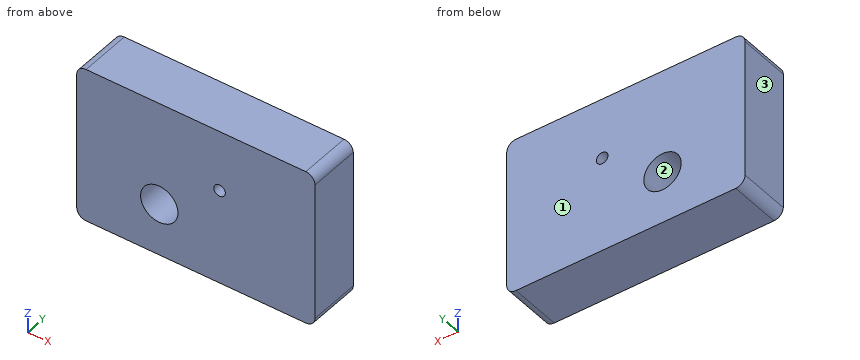
```python
from build123d import *

# Parameters (mm, degrees)
SKETCH1_W           = 27.5
SKETCH1_H           = 18
SKETCH1_R           = 2.25
SKETCH1_R_2         = 0.75
BOSS_EXTRUDE1_DEPTH = 6
FILLET1_R           = 1
MOVE_FACE1_BY       = 0.08
MOVE_FACE1_2_BY     = 0.08
MOVE_FACE1_3_BY     = 0.08
MOVE_FACE1_4_BY     = 0.08
MOVE_FACE1_5_BY     = 0.08
MOVE_FACE1_6_BY     = 0.08
MOVE_FACE1_7_BY     = 0.08
MOVE_FACE1_8_BY     = 0.08
MOVE_FACE1_9_BY     = 0.08
MOVE_FACE1_10_BY    = 0.08


with BuildPart() as part:
    # Sketch1 → Boss-Extrude1 (new body)
    with BuildSketch(Plane(origin=(0, 0, 0), x_dir=(1, 0, 0), z_dir=(0, 1, 0))):
        with Locations((13.75, 9)):
            Rectangle(SKETCH1_W, SKETCH1_H)
        with Locations(Location((9.5, 12, 0), (0, 0, 270))):
            Circle(SKETCH1_R, mode=Mode.SUBTRACT)
        with Locations(Location((16.5, 7, 0), (0, 0, 270))):
            Circle(SKETCH1_R_2, mode=Mode.SUBTRACT)
    extrude(amount=BOSS_EXTRUDE1_DEPTH)

    # Fillet1
    fillet1_edges = [part.edges().sort_by_distance(p)[0] for p in [
        (0, 3, -18),
        (27.5, 3, -18),
        (27.5, 3, 0),
        (0, 3, 0),
    ]]
    fillet(fillet1_edges, radius=FILLET1_R)

    # Move Face1: a curved face moved outward by 0.08
    add(Solid.thicken(part.faces().sort_by_distance((16.5, 3, -7.75))[0], MOVE_FACE1_BY))

    # Move Face1 2: a curved face moved outward by 0.08
    add(Solid.thicken(part.faces().sort_by_distance((9.5, 3, -14.25))[0], MOVE_FACE1_2_BY))

    # Move Face1 3: a curved face moved outward by 0.08
    add(Solid.thicken(part.faces().sort_by_distance((0.292893219, 3, -0.292893219))[0], MOVE_FACE1_3_BY))

    # Move Face1 4: a face moved outward by 0.08
    extrude(part.faces().sort_by_distance((0, 3, -9))[0], amount=MOVE_FACE1_4_BY, dir=(-1, 0, 0))

    # Move Face1 5: a curved face moved outward by 0.08
    add(Solid.thicken(part.faces().sort_by_distance((0.292893219, 3, -17.707106781))[0], MOVE_FACE1_5_BY))

    # Move Face1 6: a face moved outward by 0.08
    extrude(part.faces().sort_by_distance((13.75, 3, -18))[0], amount=MOVE_FACE1_6_BY, dir=(0, 0, -1))

    # Move Face1 7: a curved face moved outward by 0.08
    add(Solid.thicken(part.faces().sort_by_distance((27.207106781, 3, -17.707106781))[0], MOVE_FACE1_7_BY))

    # Move Face1 8: a face moved outward by 0.08
    extrude(part.faces().sort_by_distance((27.5, 3, -9))[0], amount=MOVE_FACE1_8_BY, dir=(1, 0, 0))

    # Move Face1 9: a curved face moved outward by 0.08
    add(Solid.thicken(part.faces().sort_by_distance((27.207106781, 3, -0.292893219))[0], MOVE_FACE1_9_BY))

    # Move Face1 10: a face moved outward by 0.08
    extrude(part.faces().sort_by_distance((13.75, 3, 0))[0], amount=MOVE_FACE1_10_BY, dir=(0, 0, 1))


solid = part.part
```
The listing builds one solid part. Answer for the finished solid, in the listing's coordinates (mm). Face numbers are marked on the shaded views. Give positions to 0.01 mm unless a question says otherwise; leave off trailing zeros. Write each loop counter-clockwise with the first axis right and the second up, starting at its lowest first coordinate (ties: lowest second). Pieces come first, ordered by that corner, then holes. Notation, with made-up numbers: (73, -34.5) -> (116, -34.5) arc R9 ccw to (116, -26.5) -> close; hole circle Ø1 at (36.25, -17.5). An arc over 180 degrees is marked (long way). Write item = value, one per line. Start each with the question number.
1) Determine the mould class of the marked faces 1, 2 and 3 for opening direction X: +X half, -X half, draft (parallel to the pull), parting line (faces both ways), or undercut.
2) The part is cut by section A-A, the plane z = -7. Determine the outline of the cut face in (x, y), and give its area (3 significant figures).
3) The part is cut by section B-B, the plane y = 3.25. Determine the outline of the cut face in (x, z), and give its area (3 significant figures).
4) Straight lines are drawn through the part: line 1 along X through (y, z) = (4.3, -7); line 2 along X through (y, z) = (2.9, -12); line 3 along Z through (x, y) = (7.75, 4.95). For each, find the intervals that lie inside material, in ascending order.
5) The part is cut by section C-C, the plane x = 16.5. Determine the outline of the cut face in (y, z), and give its area (3 significant figures).
Solutions:
q1.face_1 = draft
q1.face_2 = undercut
q1.face_3 = -X half
q2.outline = (-0.08, 0) -> (15.83, 0) -> (15.83, 6) -> (-0.08, 6) -> close; (17.17, 0) -> (27.58, 0) -> (27.58, 6) -> (17.17, 6) -> close
q2.area = 158 mm²
q3.outline = (-0.08, -17) arc R1.08 ccw to (1, -18.08) -> (26.5, -18.08) arc R1.08 ccw to (27.58, -17) -> (27.58, -1) arc R1.08 ccw to (26.5, 0.08) -> (1, 0.08) arc R1.08 ccw to (-0.08, -1) -> close; hole circle Ø4.34 at (9.5, -12); hole circle Ø1.34 at (16.5, -7)
q3.area = 485 mm²
q4.line_1 = -0.08 to 15.83, 17.17 to 27.58
q4.line_2 = -0.08 to 7.33, 11.67 to 27.58
q4.line_3 = -18.08 to -13.28, -10.72 to 0.08
q5.outline = (0, -18.08) -> (6, -18.08) -> (6, -7.67) -> (0, -7.67) -> close; (0, -6.33) -> (6, -6.33) -> (6, 0.08) -> (0, 0.08) -> close
q5.area = 101 mm²
